```python
from build123d import *

# Parameters (mm, degrees)
F1_DEPTH = 50.8
F2_W     = 20.2671810985
F2_H     = 8.7723657489
F3_DEPTH = 25.4


with BuildPart() as f1:
    # F0 (on Front) → F1 (new body)
    with BuildSketch(Plane.XZ):
        Polygon((50.4421505383, 28.1019427396), (39.7014406272, 46.614386835), (18.2988387989, 46.5688812451), (7.6369468817, 28.0109315597), (18.3776567927, 9.4984874643), (39.780258621, 9.5439930542), align=None)
    extrude(amount=F1_DEPTH)

    # F2 (on Front) → F3 (join)
    with BuildSketch(Plane.XZ):
        with Locations((28.8883000612, 50.8192069829)):
            Rectangle(F2_W, F2_H)
    extrude(amount=F3_DEPTH)

    # F3_face (on face) → F4 (revolve)
    with BuildSketch(Plane(origin=(28.8798511824, -25.4, 50.8983840717), x_dir=(1, 0, 0), z_dir=(0, -1, 0))):
        Polygon((10.1420394281, 4.3070057856), (-10.1251416704, 4.3070057856), (-10.1251416704, -4.3285335675), (10.1420394281, -4.2854420762), align=None)
    revolve(axis=Axis((39.0218906105, -25.4, 50.9091659264), (0, 0, 1)))


solid = f1.part
```
CAD build for the part. Positions are in the model's coordinates, mm. A direction names the side the tool comes from. Coordinates: 2 decimals unless noted, no trailing zeros. Loops run counter-clockwise (first coordinate to the right, second up) from the corner with the lowest first, then second, coordinate; pieces in that order, holes last. Notation, with made-up numbers: (44.25, 88) - (69.25, 88) arc R27 ccw to (69.25, 122) - close; hole circle Ø10 at (3.5, 31). An arc over 180 degrees is marked (long way). Return JSON: item names as keys, results as strings.
1. Band-saw the part on A-A (x = 30.5). Give the cut face in (y, z), and give its area (3 significant figures).
Result:
{"outline": "(-50.8, 9.52) - (0, 9.52) - (0, 55.21) - (-43.79, 55.21) - (-43.79, 46.59) - (-50.8, 46.59) - close", "area": "2,260 mm2"}
2. 3-axis set-ups, long thin cutter, end or side, ignore diameter. For faces 1 (the flat face through (18.755, -13, 51)), 2 (the cylindrical face through (52.87, -40.2, 50.83)): which of +Z, -Z, +X, -X, +Y, -Y reach the whole face in a straight line?
Result:
{"face 1": "+Z, -X, +Y, -Y", "face 2": "+Z"}
3. Drop flat-ended pins along their axis: pin 1 (8 mm diameter, centred on y = -18, z = 48, fed in from +X); pin 2 (2.5 mm diameter, centred on y = -12.5, z = 51.5, fed in from -X); pin 3 (6 mm diameter, centred on y = -6, z = 46.5, fed in from -X). Give the stop position or say it passes through.
Result:
{"pin 1": "stops at x = 59", "pin 2": "stops at x = 18.75", "pin 3": "stops at x = 16.54"}
4. Probe L1, parallel to Z at x = 24, y = -41; L2, parallel to Z at x = 37, y = -38; L3, parallel to X at y = -26, z = 48. List the from-to ranges inside material, lowest first. Write a range as from..to.
Result:
{"L1": "z = 9.51..46.58", "L2": "z = 9.54..55.21", "L3": "x = 18.76..59.28"}
5. Band-saw the part on C-C (x = 14.5). Give the cut face in (y, z).
Result:
{"outline": "(-50.8, 16.18) - (0, 16.18) - (0, 39.96) - (-50.8, 39.96) - close"}
6. Mould opens along Z. For faces 3 (the flat face through (12.932, -25.044, 18.884)), 4 (the flat face through (45.147, -25.044, 37.229)), 5 (the flat face through (39, -23, 55.205)) say: released by +Z, released by -Z, zero draft, split by the parting line, or undercut.
Result:
{"face 3": "released by -Z", "face 4": "undercut", "face 5": "released by +Z"}
7. Band-saw the part on B-B (z = 49.5). Give the cut face in (x, y), and give its area (3 significant figures).
Result:
{"outline": "(18.75, -25.4) arc R20.27 ccw (long way) to (39.02, -5.13) - (39.02, 0) - (18.75, 0) - close", "area": "1,480 mm2"}
